Source: three-view drawing plus pictorial views. Frame: mm from the lowest corner of the part. Give positions to 0.01 mm unless a question says otherwise; leave off trailing zeros. Write each loop counter-clockwise with the first axis right and the second up, starting at its lowest first coordinate (ties: lowest second). Pieces come first, ordered by that corner, then holes.
Q1. Cut plane D-D on x = 119.5. Return the cut outline in (y, z), plus the area to 3 significant figures.
Q2. Cut plane C-C on z = 8.5. Return the cut outline in (x, y).
Q3. Line query: L1, parallel to Y at x = 77, z = 3.5; L2, parallel to X at y = 78.5, z = 8.75; L3, parallel to X at y = 27, z = 6.5. Output: solid intervals per line, ascending.
Q4. Cut plane A-A on x = 77. Return the cut outline in (y, z), plus the area to 3 significant figures.
Q5. Pin query (flat end, axial travel): pin 1 (4 mm diameter, centred on y = 34.5, z = 2, fed in from +X); pin 2 (5 mm diameter, centred on y = 92.5, z = 6.5, fed in from -X); pin 3 (3 mm diameter, centred on y = 101.5, z = 5.5, fed in from -X). Return the tip coordinate at first contact, or that it passes through.
Q6. Cut plane B-B on y = 127. Return the cut outline in (x, z), plus the area to 3 significant figures.
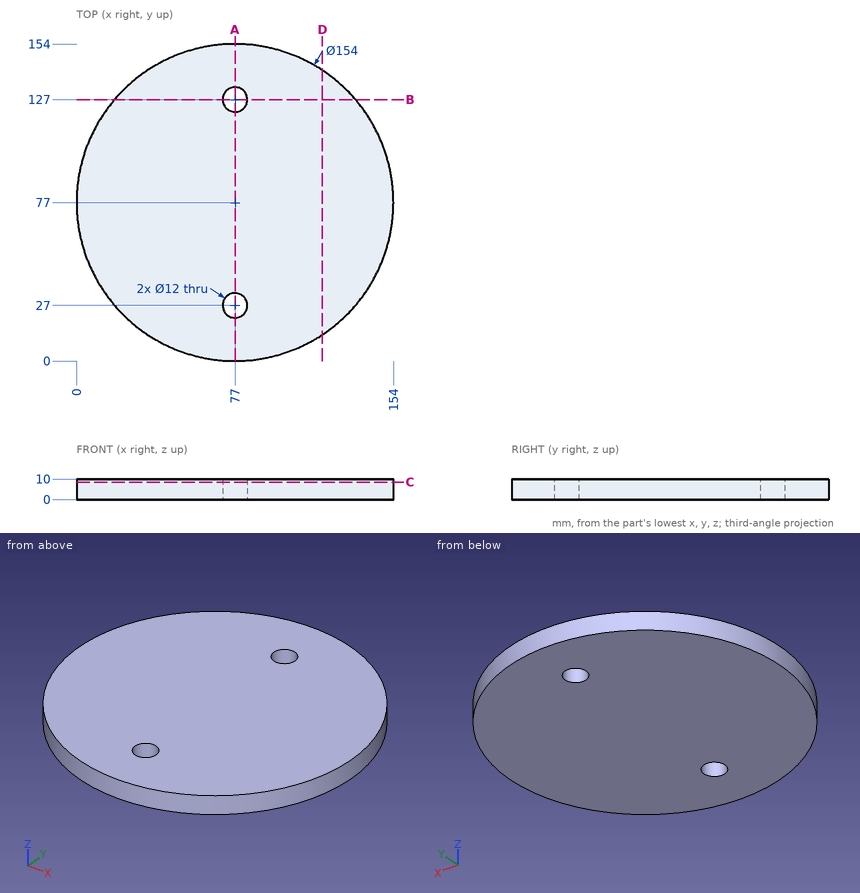
Data:
1. outline: (12.79, 0) - (141.21, 0) - (141.21, 10) - (12.79, 10) - close
1. area: 1,280 mm2
2. outline: circle Ø154 at (77, 77); hole circle Ø12 at (77, 27); hole circle Ø12 at (77, 127)
3. L1: y = 0 to 21, 33 to 121, 133 to 154
3. L2: x = 0.01 to 153.99
3. L3: x = 18.44 to 71, 83 to 135.56
4. outline: (0, 0) - (21, 0) - (21, 10) - (0, 10) - close; (33, 0) - (121, 0) - (121, 10) - (33, 10) - close; (133, 0) - (154, 0) - (154, 10) - (133, 10) - close
4. area: 1,300 mm2
5. pin 1: stops at x = 142.49
5. pin 2: stops at x = 1.11
5. pin 3: stops at x = 3.52
6. outline: (18.44, 0) - (71, 0) - (71, 10) - (18.44, 10) - close; (83, 0) - (135.56, 0) - (135.56, 10) - (83, 10) - close
6. area: 1,050 mm2
